Design review of the part shown in the three views and the two pictorial views. Dimensions are in mm from the part's minimum x, y and z. A direction names the side the tool comes from. Coordinates: 2 decimals unless noted, no trailing zeros. Write each loop counter-clockwise with the first axis right and the second up, starting at its lowest first coordinate (ties: lowest second). Pieces come first, ordered by that corner, then holes.
Q1. Take a section at D-D, the plane x = 53. Write out the cut boundary in (y, z), plus the area to 3 significant figures.
Q2. Take a section at A-A, the plane z = 32. Write out the cut boundary in (x, y), plus the area to 3 significant figures.
Q3. For the marked faces 1, 2 and 3, list the 3-axis set-ups (+Z, -Z, +X, -X, +Y, -Y) from which the entire face can be reached by the end or side of a thin tool; tool diameter is ignored.
Q4. The part is to be moulded in two halves that separate along X. For the marked faces 4, 5 and 6, say which applies: released by +X, released by -X, zero draft, split by the parting line, or undercut.
Q5. For L1, parallel to X at y = 50.5, z = 44.5; L2, parallel to Z at x = 53, y = 45; L3, parallel to Y at x = 71, z = 36, list the stretches that pass through material, from the lowest coordinate up.
Q6. Take a section at C-C, the plane x = 11.5. Write out the cut boundary in (y, z), plus the area to 3 significant figures.
Q7. Take a section at B-B, the plane y = 44.5. Write out the cut boundary in (x, z), plus the area to 3 significant figures.
Q8. For pin 1 Ø12.5 at (x, z) = (73, 40) entering from -Y; pin 2 Ø12 at (x, y) = (45.5, 26.5) entering from +Z, all flat-tipped, find the tip position at first contact; note any pin that passes through.
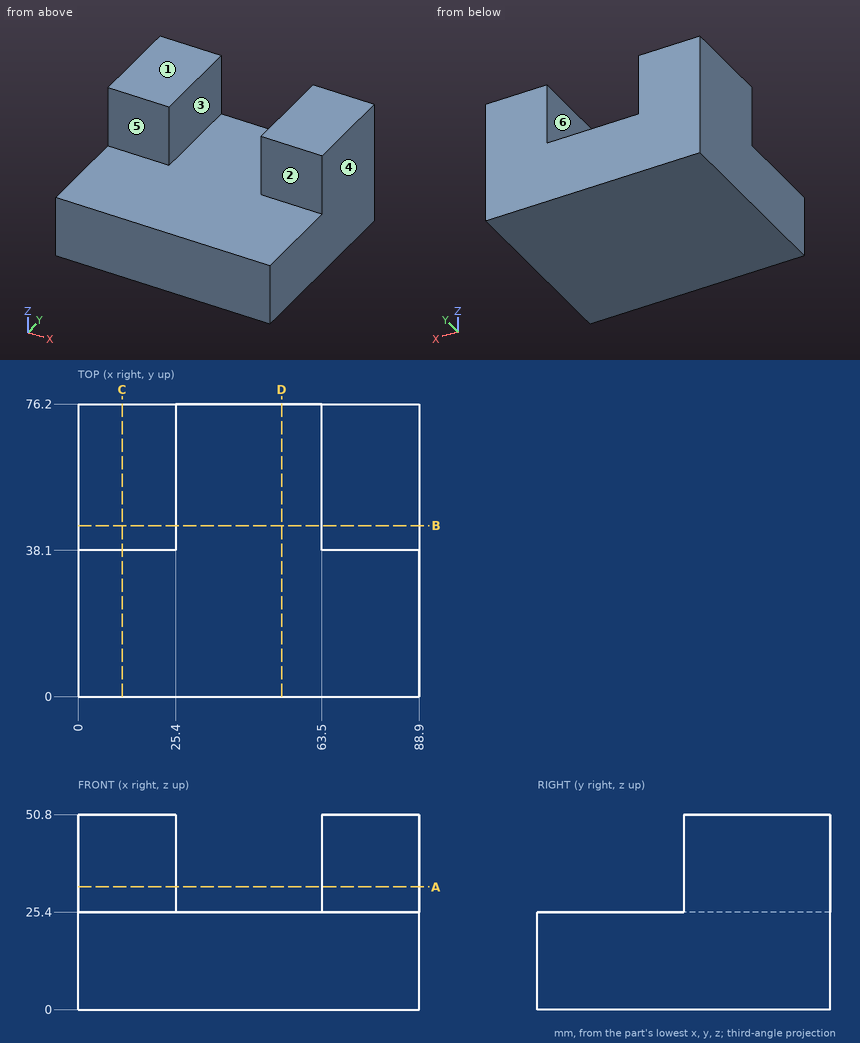
Responses:
1. outline: (0, 0) - (76.2, 0) - (76.2, 25.4) - (0, 25.4) - close
1. area: 1,940 mm2
2. outline: (0, 38.1) - (25.4, 38.1) - (25.4, 76.2) - (0, 76.2) - close; (63.5, 38.1) - (88.9, 38.1) - (88.9, 76.2) - (63.5, 76.2) - close
2. area: 1,940 mm2
3. face 1: +Z, +X, -X, +Y, -Y
3. face 2: +Z, +X, -X, -Y
3. face 3: +Z, +Y, -Y
4. face 4: released by +X
4. face 5: zero draft
4. face 6: undercut
5. L1: x = 0 to 25.4, 63.5 to 88.9
5. L2: z = 0 to 25.4
5. L3: y = 38.1 to 76.2
6. outline: (0, 0) - (76.2, 0) - (76.2, 50.8) - (38.1, 50.8) - (38.1, 25.4) - (0, 25.4) - close
6. area: 2,900 mm2
7. outline: (0, 0) - (88.9, 0) - (88.9, 50.8) - (63.5, 50.8) - (63.5, 25.4) - (25.4, 25.4) - (25.4, 50.8) - (0, 50.8) - close
7. area: 3,550 mm2
8. pin 1: stops at y = 38.1
8. pin 2: stops at z = 25.4
